Design review of the part built by this model. Coordinates are the model's own, in mm. A direction names the side the tool comes from. Coordinates: 2 decimals unless noted, no trailing zeros. Loops run counter-clockwise (first coordinate to the right, second up) from the corner with the lowest first, then second, coordinate; pieces in that order, holes last. Notation, with made-up numbers: (-8.75, -22) -> (49.25, -22) arc R19 cw to (49.25, 7) -> close; hole circle Ø9 at (4, -3). An arc over 180 degrees is marked (long way). One line per item, written item: value. Start each with the question number.
1. Insertion check: pin 1 (16.5 mm diameter, centred on x = 129.5, y = 64, fed in from +Z); pin 2 (6 mm diameter, centred on x = 9, y = 61.5, fed in from +Z); pin 3 (3 mm diameter, centred on y = 116.5, z = 4, fed in from +X); pin 4 (4 mm diameter, centred on x = 59.5, y = 120.5, fed in from -Z). Each pin has a flat end and moves straight along its axis. Give the tip position at first contact, or say it passes through.
2. Machinability: for faces 1 (the flat face through (10, 96, 2)), 2 (the flat face through (114.5, 94, 4)), 3 (the flat face through (67, 96, 0)), which of the approach directions +Z, -Z, +X, -X, +Y, -Y give a long, thin tool a straight path to every point of the face, cutting with its end or side? Answer none if there is none.
3. Add section C-C on x = 15. Write out the cut boundary in (y, z), plus the area to 3 significant figures.
4. Add section A-A on y = 29. Write out the cut boundary in (x, z), plus the area to 3 significant figures.
5. Add section B-B on z = 3.65. Write out the cut boundary in (x, y), plus the area to 3 significant figures.
6. Add section D-D on y = 118. Write out the cut boundary in (x, z), plus the area to 3 significant figures.
7. For probe 1 along Y at (x, z) = (120.5, 1.5); probe 2 along X at (y, z) = (157, 5); probe 3 along Z at (x, y) = (6.5, 11), list the stretches that pass through material, from the lowest coordinate up.
```python
from build123d import *

# Parameters (mm, degrees)
PAD_DEPTH    = 2
SKETCH004_W  = 94
SKETCH004_H  = 190
PAD001_DEPTH = 6


with BuildPart() as part:
    # Sketch001 → Pad (new body)
    with BuildSketch(Plane.XY):
        Polygon((0, 0), (135, 0), (135, 40), (115, 40), (115, 150), (135, 150), (135, 190), (0, 190), align=None)
    extrude(amount=PAD_DEPTH)

    # Sketch004 → Pad001 (join)
    with BuildSketch(Plane.XY):
        with Locations((67.5, 95)):
            Rectangle(SKETCH004_W, SKETCH004_H)
    extrude(amount=PAD001_DEPTH)


solid = part.part
```
Worked answers:
1. pin 1: passes through
1. pin 2: stops at z = 2
1. pin 3: stops at x = 114.5
1. pin 4: stops at z = 0
2. face 1: +Z, -X, +Y, -Y
2. face 2: +Z, +X, +Y, -Y
2. face 3: -Z, +X, -X, +Y, -Y
3. outline: (0, 0) -> (190, 0) -> (190, 2) -> (0, 2) -> close
3. area: 380 mm²
4. outline: (0, 0) -> (135, 0) -> (135, 2) -> (114.5, 2) -> (114.5, 6) -> (20.5, 6) -> (20.5, 2) -> (0, 2) -> close
4. area: 646 mm²
5. outline: (20.5, 0) -> (114.5, 0) -> (114.5, 190) -> (20.5, 190) -> close
5. area: 17,900 mm²
6. outline: (0, 0) -> (115, 0) -> (115, 2) -> (114.5, 2) -> (114.5, 6) -> (20.5, 6) -> (20.5, 2) -> (0, 2) -> close
6. area: 606 mm²
7. probe 1: y = 0 to 40, 150 to 190
7. probe 2: x = 20.5 to 114.5
7. probe 3: z = 0 to 2
